For this review, take the finished solid that the model builds, in its own axes (mm). Face numbers are marked on the shaded views. Give positions to 0.01 mm unless a question says otherwise; leave off trailing zeros. Order: outer loops, then holes, each group sorted by start corner. A loop starts at its lowest first (then second) coordinate and runs counter-clockwise, first axis right, second up. Notation, with made-up numbers: (32, -16) -> (64, -16) arc R33 ccw to (64, 15) -> close; hole circle Ø2 at (-26, 54.25). An arc over 180 degrees is marked (long way). Return JSON: item names as keys, results as strings. Group by question number.
1) Add section B-B (z = 4.25). Give the boundary of the cut face in (x, y).
2) Insertion check: P1, Ø1, axis at x = 2.5, y = -1, coming from the +Z side. The pin has a flat end and moves straight along its axis. Give the tip position at first contact, or say it passes through.
3) Add section C-C (y = 0.25). Give the boundary of the cut face in (x, z).
4) To check wall thickness, follow line 1 along Y through (x, z) = (0, 5); line 2 along Y through (x, z) = (2.75, 5.25); line 3 along X through (y, z) = (-0.75, 5.25). State the ranges of each line that lie inside material, in increasing order.
5) The part is to be moulded in two halves that separate along Y. For the marked faces 1, 2 and 3, say which applies: released by +Y, released by -Y, zero draft, split by the parting line, or undercut.
6) Add section A-A (x = 0). Give the boundary of the cut face in (y, z), then the cut area to 3 significant figures.
7) Add section D-D (y = 4.75). Give the boundary of the cut face in (x, z), then the cut area to 3 significant figures.
from build123d import *

# Parameters (mm, degrees)
SKETCH_1_R      = 4
EXTRUDE_1_DEPTH = 6.8
CHAMFER_1_SIZE  = 0.75


with BuildPart() as part:
    # Эскиз1 → Бобышка-Вытянуть1 (new body)
    with BuildSketch(Plane.XY):
        Polygon((3.75277675, -6.5), (7.505553499, 0), (3.75277675, 6.5), (-3.75277675, 6.5), (-7.505553499, 0), (-3.75277675, -6.5), align=None)
        Circle(SKETCH_1_R, mode=Mode.SUBTRACT)
    extrude(amount=EXTRUDE_1_DEPTH)

    # Фаска1
    chamfer_1_edges = [part.edges().sort_by_distance(p)[0] for p in [
        (5.629165125, 3.25, 6.8),
        (0, 6.5, 6.8),
        (-5.629165125, 3.25, 6.8),
        (-5.629165125, -3.25, 6.8),
        (0, -6.5, 6.8),
        (-5.629165125, -3.25, 0),
        (-5.629165125, 3.25, 0),
        (0, 6.5, 0),
        (5.629165125, 3.25, 0),
        (5.629165125, -3.25, 0),
        (0, -6.5, 0),
        (5.629165125, -3.25, 6.8),
    ]]
    chamfer(chamfer_1_edges, length=CHAMFER_1_SIZE)


solid = part.part
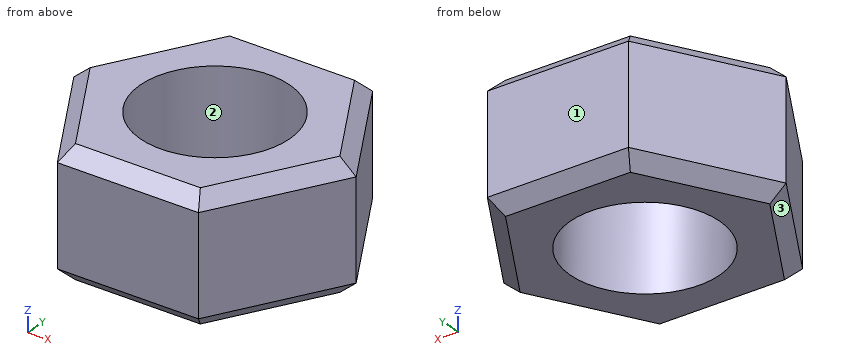
Evaluation:
{
 "1": {"outline": "(-7.51, 0) -> (-3.75, -6.5) -> (3.75, -6.5) -> (7.51, 0) -> (3.75, 6.5) -> (-3.75, 6.5) -> close; hole circle Ø8 at (0, 0)"},
 "2": {"P1": "through"},
 "3": {"outline": "(-7.36, 0.75) -> (-6.5, 0) -> (-3.99, 0) -> (-3.99, 6.8) -> (-6.5, 6.8) -> (-7.36, 6.05) -> close; (3.99, 0) -> (6.5, 0) -> (7.36, 0.75) -> (7.36, 6.05) -> (6.5, 6.8) -> (3.99, 6.8) -> close"},
 "4": {"line 1": "-6.5 to -4, 4 to 6.5", "line 2": "-6.5 to -2.9, 2.9 to 6.5", "line 3": "-7.07 to -3.93, 3.93 to 7.07"},
 "5": {"face 1": "released by +Y", "face 2": "undercut", "face 3": "released by -Y"},
 "6": {"outline": "(-6.5, 0.75) -> (-5.75, 0) -> (-4, 0) -> (-4, 6.8) -> (-5.75, 6.8) -> (-6.5, 6.05) -> close; (4, 0) -> (5.75, 0) -> (6.5, 0.75) -> (6.5, 6.05) -> (5.75, 6.8) -> (4, 6.8) -> close", "area": "32.9 mm^2"},
 "7": {"outline": "(-4.76, 0.75) -> (-3.9, 0) -> (3.9, 0) -> (4.76, 0.75) -> (4.76, 6.05) -> (3.9, 6.8) -> (-3.9, 6.8) -> (-4.76, 6.05) -> close", "area": "63.5 mm^2"}
}
